from build123d import *

# Parameters (mm, degrees)
SKETCH1_R           = 95.25
SKETCH1_R_2         = 86.487
BOSS_EXTRUDE1_DEPTH = 12.7
SKETCH3_R           = 1.7272
CUT_EXTRUDE2_DEPTH  = 254
CIRPATTERN1_COUNT   = 12


with BuildPart() as part:
    # Sketch1 → Boss-Extrude1 (new body)
    with BuildSketch(Plane(origin=(0, 0, 0), x_dir=(1, 0, 0), z_dir=(0, 1, 0))):
        Circle(SKETCH1_R)
        Circle(SKETCH1_R_2, mode=Mode.SUBTRACT)
    extrude(amount=BOSS_EXTRUDE1_DEPTH)

    # Sketch3 → Cut-Extrude2 (cut)
    with BuildSketch(Plane.XY):
        with Locations((0, 6.35)):
            Circle(SKETCH3_R)
    cut_extrude2 = extrude(amount=-CUT_EXTRUDE2_DEPTH, mode=Mode.SUBTRACT)

    # CirPattern1: Cut-Extrude2 ×12 about axis
    cirpattern1_axis = Axis((0, 12.7, 0), (0, 1, 0))
    for i in range(1, CIRPATTERN1_COUNT):
        add(cut_extrude2.rotate(cirpattern1_axis, i * 360 / CIRPATTERN1_COUNT), mode=Mode.SUBTRACT)


solid = part.part
Geometry: final body of the model. Coordinates: model frame, mm. Give positions to 0.01 mm unless a question says otherwise; leave off trailing zeros. Order: outer loops, then holes, each group sorted by start corner. A loop starts at its lowest first (then second) coordinate and runs counter-clockwise, first axis right, second up. Notation, with made-up numbers: (60.5, -40) - (101.5, -40) arc R25 cw to (101.5, -18) - close; hole circle Ø5 at (24, 60). An arc over 180 degrees is marked (long way). Use CSV: the item, a comma, the result in double quotes.
1. Section query B-B (z = 22.5). Output: boundary loops of the cut face in (x, y).
Answers below:
outline,"(-92.55, 0) - (-83.51, 0) - (-83.51, 12.7) - (-92.55, 12.7) - close; (83.51, 0) - (92.55, 0) - (92.55, 12.7) - (83.51, 12.7) - close"
2. Mould query, pull axis Z, two halves, no side actions, for faces 1 (the face through (20.7, 12.7, 84.2)), 2 (the face through (77.81, 6.869, 46.826)), 3 (the face through (-75.587, 6.261, 57.958)). Classes: +Z half, -Z half, draft (parallel to the pull), parting line (faces both ways), or undercut.
Answers below:
face 1,"draft"
face 2,"undercut"
face 3,"parting line"
3. Material intervals for line 1 along Y through (x, z) = (88.75, 0); line 2 along Z through (x, y) = (-54.5, 5.75); line 3 along X through (y, z) = (5, -41), sorted ascending. Write a range as from..to.
Answers below:
line 1,"0..4.62, 8.08..12.7"
line 2,"-78.12..-67.15, 67.15..78.12"
line 3,"-85.97..-76.15, 76.15..85.97"
4. Contact query for flat-ended pins moving along their axis: pin 1 (1 mm diameter, centred on x = 23, y = 8, fed in from -Z); pin 2 (3 mm diameter, centred on x = 20, y = 3.5, fed in from +Z); pin 3 (2 mm diameter, centred on y = 6.35, z = 0, fed in from -X); pin 4 (5 mm diameter, centred on y = 8, z = -32, fed in from +X). Output: stop coordinate, or through.
Answers below:
pin 1,"z = -92.55"
pin 2,"z = 93.44"
pin 3,"through"
pin 4,"x = 90.57"
5. Section query A-A (x = -12.5). Output: boundary loops of the cut face in (y, z).
Answers below:
outline,"(0, -94.43) - (12.7, -94.43) - (12.7, -85.58) - (0, -85.58) - close; (0, 85.58) - (12.7, 85.58) - (12.7, 94.43) - (0, 94.43) - close"
6. Section query C-C (y = 10). Output: boundary loops of the cut face in (x, z).
Answers below:
outline,"circle Ø190.5 at (0, 0); hole circle Ø172.97 at (0, 0)"
